from build123d import *

# Parameters (mm, degrees)
SKETCH1_R           = 4
SKETCH1_R_2         = 1.5
BOSS_EXTRUDE1_DEPTH = 1.5
CUT_EXTRUDE1_START  = -0.5
SKETCH2_R           = 3.5
SKETCH2_R_2         = 2
CUT_EXTRUDE1_DEPTH  = 7.903124237


with BuildPart() as part:
    # Sketch1 → Boss-Extrude1 (new, symmetric)
    with BuildSketch(Plane.XY):
        Circle(SKETCH1_R)
        Circle(SKETCH1_R_2, mode=Mode.SUBTRACT)
    extrude(amount=BOSS_EXTRUDE1_DEPTH, both=True)

    # Sketch2 → Cut-Extrude1 (cut)
    with BuildSketch(Plane.XY.offset(1.5).offset(CUT_EXTRUDE1_START)):
        with Locations(Location((0, 0, 0), (0, 0, 180))):
            Circle(SKETCH2_R)
        with Locations(Location((0, 0, 0), (0, 0, 180))):
            Circle(SKETCH2_R_2, mode=Mode.SUBTRACT)
    cut_extrude1 = extrude(amount=CUT_EXTRUDE1_DEPTH, mode=Mode.SUBTRACT)

    # Mirror1: Cut-Extrude1 across plane
    add(cut_extrude1.mirror(Plane.XY), mode=Mode.SUBTRACT)


solid = part.part
Read the model definition and answer for the solid it produces. Units are mm, in the model's axes. A direction names the side the tool comes from. Round coordinates to 2 decimals unless told otherwise and drop trailing zeros. Loops run counter-clockwise (first coordinate to the right, second up) from the corner with the lowest first, then second, coordinate; pieces in that order, holes last.
Q1. Section A-A on x = 0 is taken. Write down the section's boundary in (y, z).
Q2. Which of the six approach directions +Z, -Z, +X, -X, +Y, -Y give full straight-line access (tool end or side, diameter ignored) to faces 1 (the face through (-1.5, 0.07, -0.02)), 2 (the face through (-2, 2, -1)), 3 (the face through (-3.233, 1.341, 1.246))?
Q3. Consider probe 1 along Y at (x, z) = (0, -1.3); probe 2 along Y at (x, z) = (0, 0.9); probe 3 along Z at (x, y) = (1.5, 3). Determine where each line is inside the solid, lowest interval first.
Q4. Section B-B on z = -1.2 is taken. Write down the section's boundary in (x, y).
Q5. Determine the mould class of faces 4 (the face through (0.434, 1.952, -1.246)), 5 (the face through (-0.867, -3.905, 0.021)), 6 (the face through (-3.233, 1.341, -1.246)) for opening direction X: released by +X, released by -X, zero draft, split by the parting line, or undercut.
Q6. Section D-D on y = -3.25 is taken. Write down the section's boundary in (x, z).
Q7. This flat-tipped pin is pushed along its axis until it touches: pin 1 (1.5 mm diameter, centred on x = 2.5, z = 1, fed in from +Y). Where does it stop, or does it pass through?
Output:
1. outline: (-4, -1.5) - (-3.5, -1.5) - (-3.5, -1) - (-2, -1) - (-2, -1.5) - (-1.5, -1.5) - (-1.5, 1.5) - (-2, 1.5) - (-2, 1) - (-3.5, 1) - (-3.5, 1.5) - (-4, 1.5) - close; (1.5, -1.5) - (2, -1.5) - (2, -1) - (3.5, -1) - (3.5, -1.5) - (4, -1.5) - (4, 1.5) - (3.5, 1.5) - (3.5, 1) - (2, 1) - (2, 1.5) - (1.5, 1.5) - close
2. face 1: +Z, -Z
2. face 2: -Z
2. face 3: +Z
3. probe 1: y = -4 to -3.5, -2 to -1.5, 1.5 to 2, 3.5 to 4
3. probe 2: y = -4 to -1.5, 1.5 to 4
3. probe 3: z = -1 to 1
4. outline: circle Ø8 at (0, 0); circle Ø4 at (0, 0); hole circle Ø7 at (0, 0); hole circle Ø3 at (0, 0)
5. face 4: undercut
5. face 5: split by the parting line
5. face 6: undercut
6. outline: (-2.33, -1.5) - (-1.3, -1.5) - (-1.3, -1) - (1.3, -1) - (1.3, -1.5) - (2.33, -1.5) - (2.33, 1.5) - (1.3, 1.5) - (1.3, 1) - (-1.3, 1) - (-1.3, 1.5) - (-2.33, 1.5) - close
7. pin 1: stops at y = 3.6
